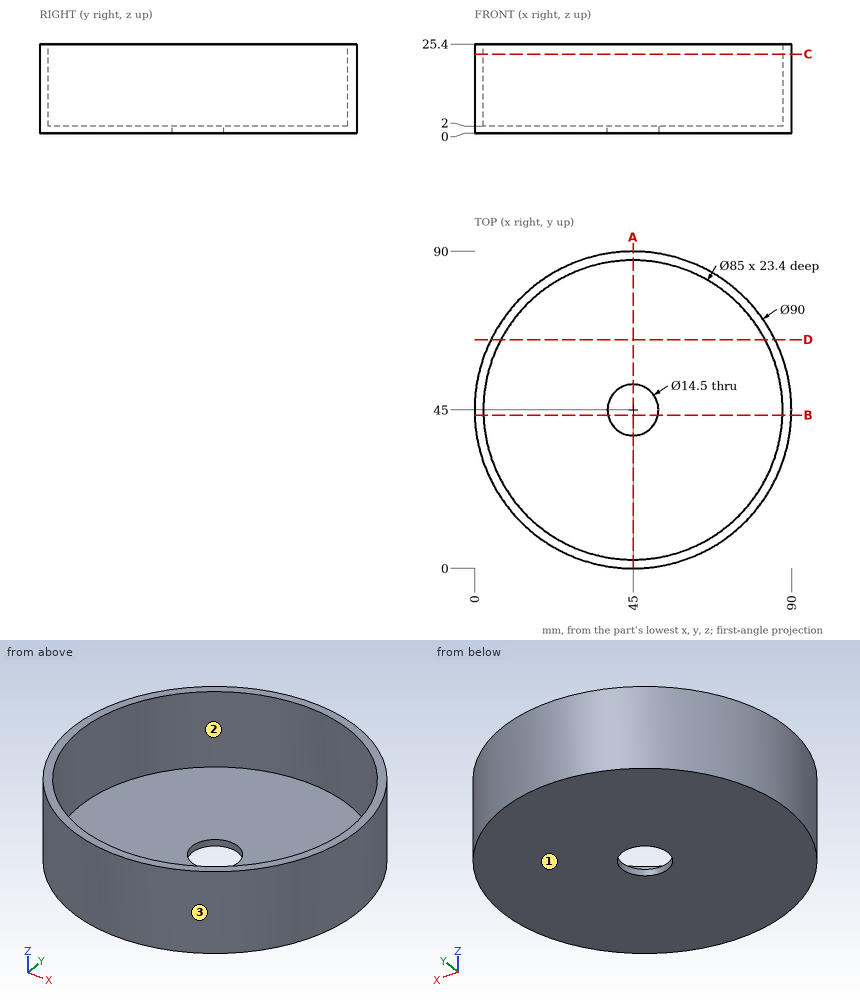
The figure shows three views and two pictorial views of one solid part (mm, origin at its lowest corner). Answer the questions. Give positions to 0.01 mm unless a question says otherwise; leave off trailing zeros. Order: outer loops, then holes, each group sorted by start corner. A loop starts at its lowest first (then second) coordinate and runs counter-clockwise, first axis right, second up. Notation, with made-up numbers: (-4, 53.25) -> (50, 53.25) arc R19 ccw to (50, 61.25) -> close; hole circle Ø4 at (-16.75, 61.25). An arc over 180 degrees is marked (long way). Answer as CSV lines item,"result". Start each with the question number.
(1) For a pull along X with two mould halves and no side action, classify the marked faces 1, 2 and 3 as released by +X, released by -X, zero draft, split by the parting line, or undercut.
(2) Section C-C, the plane z = 22.5 is taken. Write down the section's boundary in (x, y).
(3) Consider line 1 along Z through (x, y) = (33, 23); line 2 along Y through (x, z) = (45, 1.35); line 3 along X through (y, z) = (73.5, 10). Determine where each line is inside the solid, lowest interval first.
(4) Section D-D, the plane y = 65 is taken. Write down the section's boundary in (x, z), plus the area to 3 significant figures.
(5) Each of these flat-tipped pins is pushed along its axis until it touches: pin 1 Ø23 at (x, y) = (45, 45) entering from +Z; pin 2 Ø8 at (y, z) = (39, 9.5) entering from -X; pin 3 Ø3 at (y, z) = (33.5, 11.5) entering from +X. Where does it stop, or does it pass through?
(6) Section B-B, the plane y = 43.5 is taken. Write down the section's boundary in (x, z) (3 decimals), plus the area to 3 significant figures.
(7) Section A-A, the plane x = 45 is taken. Write down the section's boundary in (y, z).
Entries:
1,face 1,"zero draft"
1,face 2,"undercut"
1,face 3,"split by the parting line"
2,outline,"circle Ø90 at (45, 45); hole circle Ø85 at (45, 45)"
3,line 1,"0 to 2"
3,line 2,"0 to 37.75, 52.25 to 90"
3,line 3,"10.18 to 13.47, 76.53 to 79.82"
4,outline,"(4.69, 0) -> (85.31, 0) -> (85.31, 25.4) -> (82.5, 25.4) -> (82.5, 2) -> (7.5, 2) -> (7.5, 25.4) -> (4.69, 25.4) -> close"
4,area,"293 mm²"
5,pin 1,"z = 2"
5,pin 2,"x = 0.04"
5,pin 3,"x = 88.87"
6,outline,"(0.025, 0) -> (37.907, 0) -> (37.907, 2) -> (2.526, 2) -> (2.526, 25.4) -> (0.025, 25.4) -> close; (52.093, 0) -> (89.975, 0) -> (89.975, 25.4) -> (87.474, 25.4) -> (87.474, 2) -> (52.093, 2) -> close"
6,area,"269 mm²"
7,outline,"(0, 0) -> (37.75, 0) -> (37.75, 2) -> (2.5, 2) -> (2.5, 25.4) -> (0, 25.4) -> close; (52.25, 0) -> (90, 0) -> (90, 25.4) -> (87.5, 25.4) -> (87.5, 2) -> (52.25, 2) -> close"
